from build123d import *

# Parameters (mm, degrees)
BOSS_EXTRUDE1_DEPTH                              = 22.225
SKETCH2_W                                        = 3.683
SKETCH2_H                                        = 3.683
BOSS_EXTRUDE2_DEPTH                              = 101.6
CUT_EXTRUDE1_DEPTH                               = 108.059192156
FILLET1_R                                        = 2.54
CSK_FOR_1_4_FLAT_HEAD_MACHINE_SCREW1_D           = 7.14248
CSK_FOR_1_4_FLAT_HEAD_MACHINE_SCREW1_CSINK_D     = 13.7609834
CSK_FOR_1_4_FLAT_HEAD_MACHINE_SCREW1_CSINK_ANGLE = 82
CUT_EXTRUDE2_DEPTH                               = 106.732743864
FILLET2_R                                        = 2.54
CHAMFER1_SIZE                                    = 3.683


with BuildPart() as part:
    # Sketch1 → Boss-Extrude1 (new, symmetric)
    with BuildSketch(Plane(origin=(0, 0, 0), x_dir=(1, 0, 0), z_dir=(0, 1, 0))):
        Polygon((0, 0), (0, 101.6), (-6.35, 101.6), (-6.35, 4.7625), (-25.4, 4.7625), (-25.4, 0), align=None)
    extrude(amount=BOSS_EXTRUDE1_DEPTH, both=True)

    # Sketch2 → Boss-Extrude2 (add)
    with BuildSketch(Plane.XY):
        with Locations((1.8415, 20.3835)):
            Rectangle(SKETCH2_W, SKETCH2_H)
        with Locations((1.8415, -20.3835)):
            Rectangle(SKETCH2_W, SKETCH2_H)
    extrude(amount=-BOSS_EXTRUDE2_DEPTH)

    # Sketch3 → Cut-Extrude1 (cut, through all)
    with BuildSketch(Plane.XY):
        with BuildLine():
            Line((-17.33005, 19.1262), (-12.83245, 19.1262))
            ThreePointArc((-12.83245, 19.1262), (-9.58125, 15.875), (-12.83245, 12.6238))
            Line((-12.83245, 12.6238), (-17.33005, 12.6238))
            ThreePointArc((-17.33005, 12.6238), (-20.58125, 15.875), (-17.33005, 19.1262))
        make_face()
        with BuildLine():
            Line((-17.33005, -19.1262), (-12.83245, -19.1262))
            ThreePointArc((-12.83245, -19.1262), (-9.58125, -15.875), (-12.83245, -12.6238))
            Line((-12.83245, -12.6238), (-17.33005, -12.6238))
            ThreePointArc((-17.33005, -12.6238), (-20.58125, -15.875), (-17.33005, -19.1262))
        make_face()
    extrude(amount=-CUT_EXTRUDE1_DEPTH, mode=Mode.SUBTRACT)

    # Fillet1
    fillet1_edges = [part.edges().sort_by_distance(p)[0] for p in [
        (-25.4, 22.225, -2.38125),
        (-25.4, -22.225, -2.38125),
    ]]
    fillet(fillet1_edges, radius=FILLET1_R)

    # CSK for 1/4 Flat Head Machine Screw1 (through all)
    with Locations(Plane.ZY.offset(6.35)):
        with Locations((-19.05, 0), (-88.9, 0)):
            CounterSinkHole(CSK_FOR_1_4_FLAT_HEAD_MACHINE_SCREW1_D / 2, CSK_FOR_1_4_FLAT_HEAD_MACHINE_SCREW1_CSINK_D / 2, counter_sink_angle=CSK_FOR_1_4_FLAT_HEAD_MACHINE_SCREW1_CSINK_ANGLE)

    # Sketch6 → Cut-Extrude2 (cut, through all)
    with BuildSketch(Plane.ZY.offset(6.35)):
        Polygon((-101.6, 22.225), (-88.9, 22.225), (-101.6, 9.525), align=None)
        Polygon((-88.9, -22.225), (-101.6, -9.525), (-101.6, -22.225), align=None)
    extrude(amount=-CUT_EXTRUDE2_DEPTH, mode=Mode.SUBTRACT)

    # Fillet2
    fillet2_edges = [part.edges().sort_by_distance(p)[0] for p in [
        (-6.35, 0, -101.6),
        (-3.175, 9.525, -101.6),
        (-6.35, 15.875, -95.25),
        (-3.175, -9.525, -101.6),
        (-6.35, -15.875, -95.25),
    ]]
    fillet(fillet2_edges, radius=FILLET2_R)

    # Chamfer1
    chamfer1_edges = [part.edges().sort_by_distance(p)[0] for p in [
        (0, -18.542, -46.2915),
        (0, 18.542, -46.2915),
    ]]
    chamfer(chamfer1_edges, length=CHAMFER1_SIZE - 0.0001)  # a hair under: the kernel refuses the full size


solid = part.part
Here's how the part is built. I have some questions about the finished solid (model axes, mm). A direction names the side the tool comes from. Give positions to 0.01 mm unless a question says otherwise; leave off trailing zeros. Order: outer loops, then holes, each group sorted by start corner. A loop starts at its lowest first (then second) coordinate and runs counter-clockwise, first axis right, second up. Notation, with made-up numbers: (-26, 6) -> (18, 6) arc R15 cw to (18, 11) -> close; hole circle Ø6 at (80.5, 68.5). An arc over 180 degrees is marked (long way). One line per item, written item: value. Start each with the question number.
1. Imagine slicing it at C-C, the plane x = -15. List the corners of the cut face in (y, z) for me (1 decimal), plus the area to 3 significant figures.
2. For faces 1 (the face through (-4, 22.225, -34)), 2 (the face through (1.87, 16.73, -47.46)), 3 (the face through (-15, 12.624, -2)), which set-ups out of +Z, -Z, +X, -X, +Y, -Y let a thin tool reach every point of the face, with its end or its side?
3. Imagine slicing it at B-B, the plane y = 0. List the corners of the cut face in (x, z) for me.
4. Will these pins go through, and if not, where does the flat tip stop? pin 1 Ø6 at (y, z) = (-2.5, -25.5) entering from +X; pin 2 Ø5.5 at (x, y) = (-13.5, 0.5) entering from -Z; pin 3 Ø2 at (y, z) = (15, -65) entering from +X; pin 4 Ø1.5 at (x, z) = (-8.5, -34.5) entering from +Y.
5. We'd pull the mould along X, two halves only. Please class faces 4 (the face through (-16, 0, -4.762)), 5 (the face through (1.87, -16.73, -47.46)), 6 (the face through (-9.582, 15.946, -2.348)), 7 (the face through (-15, 19.126, -2)): released by +X, released by -X, zero draft, split by the parting line, or undercut.
6. I need wall thicknesses on probe 1 along Z at (x, y) = (-0.75, 0); probe 2 along Y at (x, z) = (-1.3, -19.05) (3 decimals); probe 3 along X at (y, z) = (6.5, -96.5). Which ranges of each line are inside material? Lowest first, please. Write a range as from..to.
Values follow:
1. outline: (-22.2, -4.8) -> (-19.1, -4.8) -> (-19.1, 0) -> (-22.2, 0) -> close; (-12.6, -4.8) -> (12.6, -4.8) -> (12.6, 0) -> (-12.6, 0) -> close; (19.1, -4.8) -> (22.2, -4.8) -> (22.2, 0) -> (19.1, 0) -> close
1. area: 150 mm2
2. face 1: +Z, -Z, +X, -X, +Y
2. face 2: +Z, -Z, +X
2. face 3: +Z, -Z
3. outline: (-25.4, -4.76) -> (-6.35, -4.76) -> (-6.35, -12.17) -> (-2.54, -15.48) -> (0, -15.48) -> (0, 0) -> (-25.4, 0) -> close; (-6.35, -99.06) arc R2.54 ccw to (-3.81, -101.6) -> (0, -101.6) -> (0, -92.47) -> (-2.54, -92.47) -> (-6.35, -95.78) -> close; (-6.35, -82.02) -> (-2.54, -85.33) -> (0, -85.33) -> (0, -22.62) -> (-2.54, -22.62) -> (-6.35, -25.93) -> close
4. pin 1: stops at x = 0
4. pin 2: stops at z = -4.76
4. pin 3: stops at x = 1.14
4. pin 4: passes through
5. face 4: zero draft
5. face 5: released by +X
5. face 6: undercut
5. face 7: undercut
6. probe 1: z = -101.6..-92.47, -85.33..-22.62, -15.48..0
6. probe 2: y = -22.225..-3.571, 3.571..22.225
6. probe 3: x = -6.35..0
